Source: three-view drawing plus pictorial views. Frame: mm from the lowest corner of the part. A direction names the side the tool comes from. Coordinates: 2 decimals unless noted, no trailing zeros. Loops run counter-clockwise (first coordinate to the right, second up) from the corner with the lowest first, then second, coordinate; pieces in that order, holes last. Notation, with made-up numbers: (34.25, 75.5) - (58.25, 75.5) arc R20 ccw to (58.25, 105.5) - close; hole circle Ø4 at (33.25, 87.5). An arc over 180 degrees is marked (long way). Return JSON: item names as keys, results as strings.
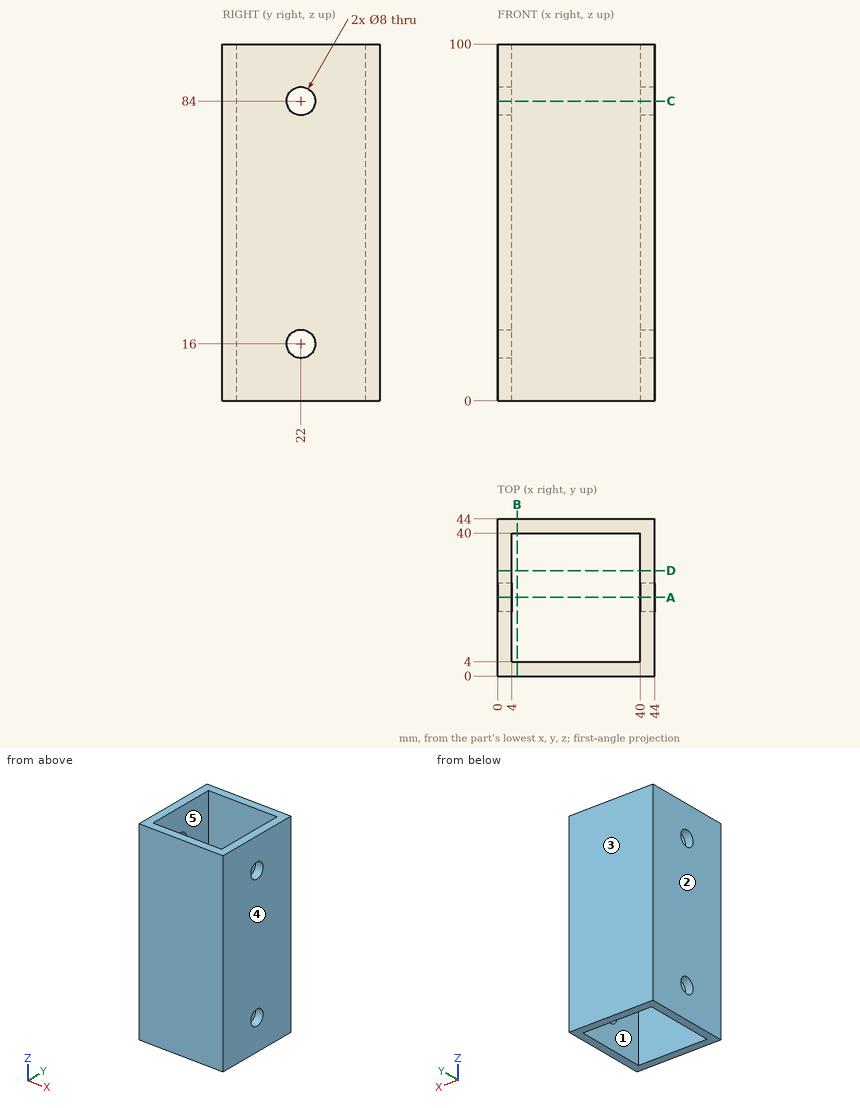
Item 1: Section query C-C, the plane z = 84. Return loops of the section in (x, y).
Worked out:
{"outline": "(0, 0) - (44, 0) - (44, 18) - (40, 18) - (40, 4) - (4, 4) - (4, 18) - (0, 18) - close; (0, 26) - (4, 26) - (4, 40) - (40, 40) - (40, 26) - (44, 26) - (44, 44) - (0, 44) - close"}
Item 2: Mould query, pull axis Y, two halves, no side actions, for the marked faces 1, 2 and 3. Classes: +Y half, -Y half, draft (parallel to the pull), parting line (faces both ways), or undercut.
Worked out:
{"face 1": "undercut", "face 2": "draft", "face 3": "+Y half"}
Item 3: First-contact query: pin 1 Ø8 at (y, z) = (13, 43) entering from -X. Flat tip, straight axial feed; report the tip coordinate or a pass-through.
Worked out:
{"pin 1": "x = 0"}
Item 4: Ray query, probe 1 along X at (y, z) = (17, 83.5); probe 2 along Y at (x, z) = (42.7, 84). Return the intervals inside material, ascending. Write a range as from..to.
Worked out:
{"probe 1": "0..4, 40..44", "probe 2": "0..18, 26..44"}
Item 5: Reachability of the marked faces 4 and 5 from +Z, -Z, +X, -X, +Y, -Y: full face, straight path, thin tool, end or side. Return the list, or none.
Worked out:
{"face 4": "+Z, -Z, +X, +Y, -Y", "face 5": "+Z, -Z"}
Item 6: Section query B-B, the plane x = 5.5. Return loops of the section in (y, z).
Worked out:
{"outline": "(0, 0) - (4, 0) - (4, 100) - (0, 100) - close; (40, 0) - (44, 0) - (44, 100) - (40, 100) - close"}
Item 7: Section query A-A, the plane y = 22. Return loops of the section in (x, z).
Worked out:
{"outline": "(0, 0) - (4, 0) - (4, 12) - (0, 12) - close; (0, 20) - (4, 20) - (4, 80) - (0, 80) - close; (0, 88) - (4, 88) - (4, 100) - (0, 100) - close; (40, 0) - (44, 0) - (44, 12) - (40, 12) - close; (40, 20) - (44, 20) - (44, 80) - (40, 80) - close; (40, 88) - (44, 88) - (44, 100) - (40, 100) - close"}
